Build history of the part. All positions in model axes, mm. Give positions to 0.01 mm unless a question says otherwise; leave off trailing zeros. Write each loop counter-clockwise with the first axis right and the second up, starting at its lowest first coordinate (ties: lowest second). Pieces come first, ordered by that corner, then holes.
from build123d import *

# Parameters (mm, degrees)
SKETCH1_R           = 0.889
SKETCH1_W           = 8.636
SKETCH1_H           = 3.556
BOSS_EXTRUDE1_DEPTH = 6.35


with BuildPart() as part:
    # Sketch1 → Boss-Extrude1 (new body)
    with BuildSketch(Plane.XY):
        Polygon((-4.005119969, -10.063655938), (-4.005119969, 0.096344062), (-14.165119969, 0.096344062), (-14.165119969, 3.652344062), (-4.005119969, 3.652344062), (-4.005119969, 38.911344062), (-80.205119969, 38.911344062), (-80.205119969, 32.561344062), (-86.555119969, 32.561344062), (-86.555119969, 26.211344062), (-80.205119969, 26.211344062), (-80.205119969, -24.588655938), (-29.405119969, -24.588655938), (-29.405119969, -30.938655938), (-4.005119969, -30.938655938), (-4.005119969, -15.063655938), (-8.005119969, -15.063655938), (-8.005119969, -10.063655938), align=None)
        with Locations((-83.380119969, 29.386344062)):
            Circle(SKETCH1_R, mode=Mode.SUBTRACT)
        with Locations((-75.125119969, -4.268655938)):
            Circle(SKETCH1_R, mode=Mode.SUBTRACT)
        with Locations((-22.505119969, -27.763655938)):
            Circle(SKETCH1_R, mode=Mode.SUBTRACT)
        with Locations((-59.885119969, -4.268655938)):
            Circle(SKETCH1_R, mode=Mode.SUBTRACT)
        with Locations((-11.625119969, 17.114344062)):
            Circle(SKETCH1_R, mode=Mode.SUBTRACT)
        with Locations((-67.505119969, -19.508655938)):
            Rectangle(SKETCH1_W, SKETCH1_H, mode=Mode.SUBTRACT)
    boss_extrude1 = extrude(amount=BOSS_EXTRUDE1_DEPTH)

    # Mirror1: Boss-Extrude1 across plane
    add(boss_extrude1.mirror(Plane(origin=(-4.005119969, -10.063655938, 6.35), x_dir=(0, 0, 1), z_dir=(-1, 0, 0))))


solid = part.part
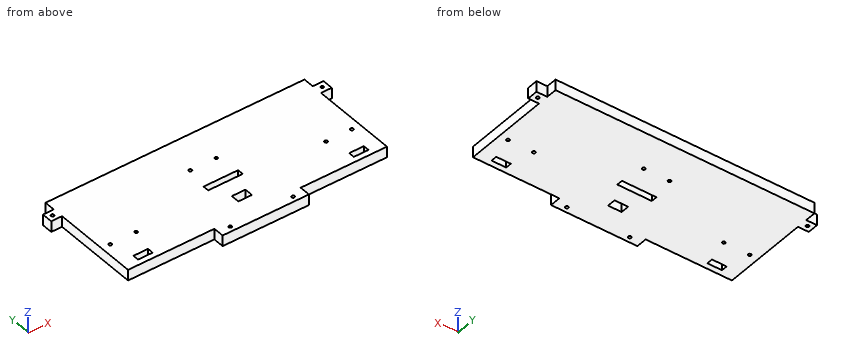
(1) Saw through at A-A, the plane y = 6.5. List the corners of the cut face in (x, z), plus the area to 3 significant figures.
(2) Saw through at B-B, the plane x = -41.5. List the corners of the cut face in (y, z), plus the area to 3 significant figures.
(3) Saw through at C-C, the plane z = 5. Give the number of separate pieces and of enclosed holes in the cut face, plus the area to 3 significant figures.
(4) Drop flat-ended pins along their axis: pin 1 (1.5 mm diameter, centred on y = 8.5, z = 5.5, fed in from -X); pin 2 (3 mm diameter, centred on x = 43.5, z = 4, fed in from -Y); pin 3 (2.5 mm diameter, centred on x = 14.49, y = -27.76, fed in from +Z); pin 4 (3 mm diameter, centred on x = 75, z = 3.5, fed in from +Y). Give the stop position or say it passes through.
(5) Probe line 1 (X direction, y = -4.5, z = 3); line 2 (Y direction, x = -9, z = 2.75); line 3 (X direction, y = -25.5, z = 4). List the from-to ranges inside material, lowest first.
Computed values:
1. outline: (-80.21, 0) - (72.19, 0) - (72.19, 6.35) - (-80.21, 6.35) - close
1. area: 968 mm2
2. outline: (-24.59, 0) - (38.91, 0) - (38.91, 6.35) - (-24.59, 6.35) - close
2. area: 403 mm2
3. separate pieces: 1
3. enclosed holes: 14
3. area: 9,880 mm2
4. pin 1: stops at x = -80.21
4. pin 2: stops at y = -24.59
4. pin 3: stops at z = 6.35
4. pin 4: stops at y = 32.56
5. line 1: x = -80.21 to -75.98, -74.27 to -60.74, -59.03 to 51.02, 52.73 to 66.26, 67.97 to 72.19
5. line 2: y = -30.94 to 0.1, 3.65 to 38.91
5. line 3: x = -29.41 to 21.39
